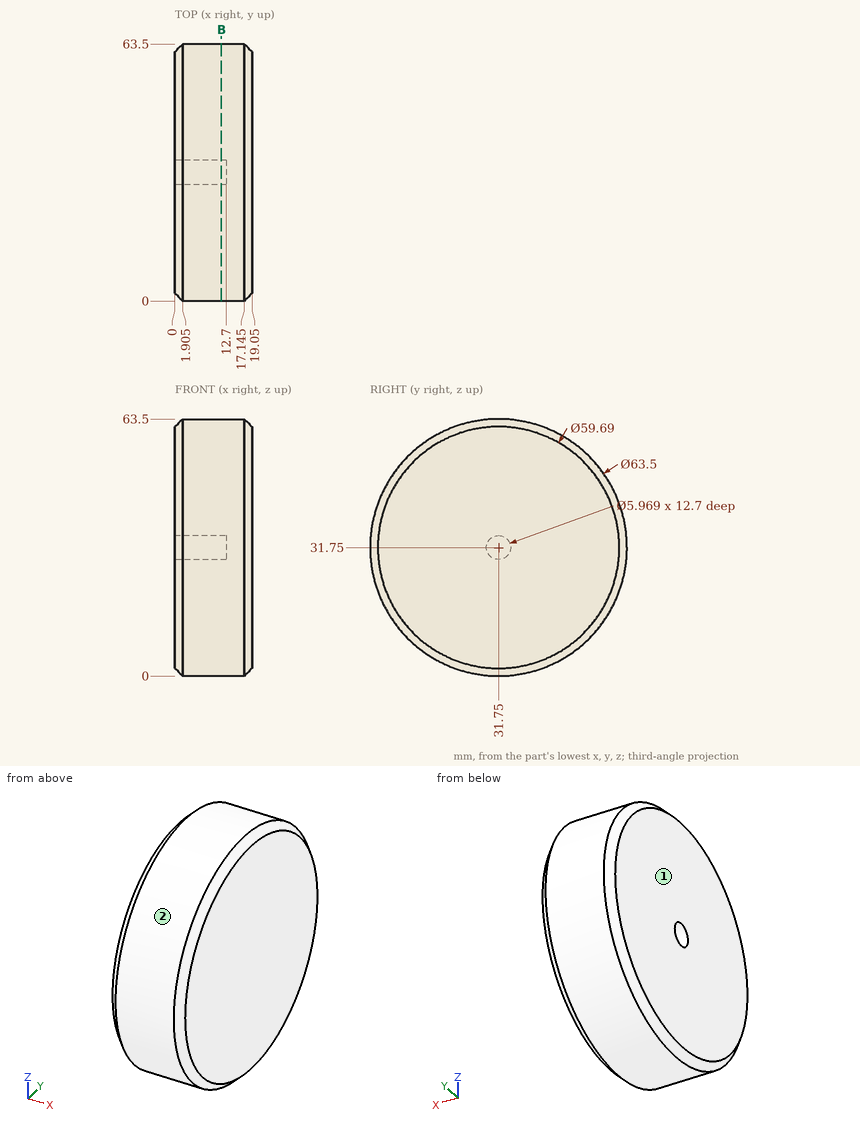
Print and shaded views of the part. All mm, measured from the part's lowest x, y and z. Round coordinates to 2 decimals unless told otherwise and drop trailing zeros. Write each loop counter-clockwise with the first axis right and the second up, starting at its lowest first coordinate (ties: lowest second). Pieces come first, ordered by that corner, then holes. Notation, with made-up numbers: (20, -30) -> (30, -30) arc R20 cw to (30, -17) -> close; hole circle Ø3 at (33, 20.25). An arc over 180 degrees is marked (long way). Write item = value, one per line.
(1) Two-plate mould, pull along Z, no slides. Class the marked faces 1 and 2: pulls with the +Z half, pulls with the -Z half, needs draft (parallel to the pull), parting line crosses it, or undercut.
Answer:
face_1 = needs draft
face_2 = parting line crosses it
(2) Band-saw the part on B-B (x = 11.5). Give the cut face in (y, z).
Answer:
outline = circle Ø63.5 at (31.75, 31.75); hole circle Ø5.97 at (31.75, 31.75)
(3) Probe L1, parallel to Z at x = 12.5, y = 32; L2, parallel to Y at x = 9.25, z = 31.75; L3, parallel to Z at x = 10.25, y = 33. List the from-to ranges inside material, lowest first.
Answer:
L1 = 0 to 28.78, 34.72 to 63.5
L2 = 0 to 28.77, 34.73 to 63.5
L3 = 0.02 to 29.04, 34.46 to 63.48
(4) Flat gauge pins, fed straight in: pin 1 (8 mm diameter, centred on x = 11, y = 45.5, fed in from -Z); pin 2 (4 mm diameter, centred on x = 13.5, z = 25.5, fed in from -Y); pin 3 (10 mm diameter, centred on x = 9.5, y = 21.5, fed in from +Z). Where does each tip first touch, or does it go through?
Answer:
pin_1 = 1.53
pin_2 = 0.29
pin_3 = 63.06
